CAD build for the part. Positions are in the model's coordinates, mm. Coordinates: 2 decimals unless noted, no trailing zeros. Loops run counter-clockwise (first coordinate to the right, second up) from the corner with the lowest first, then second, coordinate; pieces in that order, holes last. Notation, with made-up numbers: (43.25, 43.25) -> (102.25, 43.25) arc R14 ccw to (102.25, 55.25) -> close; hole circle Ø2 at (-28.5, -39.75). An arc over 180 degrees is marked (long way). Return JSON: item names as keys, results as strings. Group by question number.
(1) Saw through at A-A on z = 2.3. Write the cut outline in (x, y) (3 decimals), then the cut area to 3 significant figures.
(2) Saw through at C-C on y = -30. Write the cut outline in (x, z), then the cut area to 3 significant figures.
(3) Saw through at B-B on y = -72. Write the cut outline in (x, z), then the cut area to 3 significant figures.
(4) Flat gauge pins, fed straight in: pin 1 Ø2 at (x, y) = (44, -75.5) entering from -Z; pin 2 Ø8.5 at (x, y) = (103.24, -70.5) entering from +Z. Where does each tip first touch, or does it go through?
(5) Probe L1, parallel to X at y = -70, z = 0.95; L2, parallel to X at y = -75, z = 1.85; L3, parallel to X at y = -8, z = 0.5. List the from-to ranges inside material, lowest first.
(6) Mould opens along X. For faces 1 (the face through (10.115, -57.366, 1.479)), 2 (the face through (61, -54, 3)), 3 (the face through (98.077, -65.769, 1.521)), 4 (the face through (103.55, -53.293, 1.521)) say: pulls with the +X half, pulls with the -X half, needs draft (parallel to the pull), parting line crosses it, or undercut.
```python
from build123d import *

# Parameters (mm, degrees)
BOSS_EXTRUDE3_DEPTH = 3
SKETCH5_R           = 2.125
SKETCH5_R_2         = 7
CUT_EXTRUDE1_DEPTH  = 10
FILLET1_R           = 10
SKETCH6_R           = 2.125
CUT_EXTRUDE2_DEPTH  = 3


with BuildPart() as part:
    # Sketch4 → Boss-Extrude3 (new body)
    with BuildSketch(Plane.XY):
        Polygon((0, 0), (118.235967878, 0), (118.235967878, -110), (19.395967878, -110), align=None)
    extrude(amount=BOSS_EXTRUDE3_DEPTH)

    # Sketch5 → Cut-Extrude1 (cut)
    with BuildSketch(Plane.XY.offset(3)):
        with Locations((105.235967878, -25)):
            Circle(SKETCH5_R)
        with Locations((15.3749641, -30)):
            Circle(SKETCH5_R)
        with Locations((103.235967878, -70.5)):
            Circle(SKETCH5_R_2)
    extrude(amount=-CUT_EXTRUDE1_DEPTH, mode=Mode.SUBTRACT)

    # Fillet1
    fillet1_edges = [part.edges().sort_by_distance(p)[0] for p in [
        (0, 0, 1.5),
        (118.235967878, 0, 1.5),
        (118.235967878, -110, 1.5),
        (19.395967878, -110, 1.5),
    ]]
    fillet(fillet1_edges, radius=FILLET1_R)

    # Sketch6 → Cut-Extrude2 (cut)
    with BuildSketch(Plane.XY.offset(3)):
        with Locations((105.235967878, -52)):
            Circle(SKETCH6_R)
    extrude(amount=-CUT_EXTRUDE2_DEPTH, mode=Mode.SUBTRACT)


solid = part.part
```
Geometry results:
{
 "1": {"outline": "(2.069, -11.736) -> (17.939, -101.736) arc R10 ccw to (27.787, -110) -> (108.236, -110) arc R10 ccw to (118.236, -100) -> (118.236, -10) arc R10 ccw to (108.236, 0) -> (11.918, 0) arc R10 ccw to start; hole circle Ø4.25 at (15.375, -30); hole circle Ø14 at (103.236, -70.5); hole circle Ø4.25 at (105.236, -52); hole circle Ø4.25 at (105.236, -25)", "area": "11,700 mm²"},
 "2": {"outline": "(5.29, 0) -> (13.25, 0) -> (13.25, 3) -> (5.29, 3) -> close; (17.5, 0) -> (118.24, 0) -> (118.24, 3) -> (17.5, 3) -> close", "area": "326 mm²"},
 "3": {"outline": "(12.7, 0) -> (96.4, 0) -> (96.4, 3) -> (12.7, 3) -> close; (110.07, 0) -> (118.24, 0) -> (118.24, 3) -> (110.07, 3) -> close", "area": "276 mm²"},
 "4": {"pin 1": "z = 0", "pin 2": "through"},
 "5": {"L1": "12.34 to 96.25, 110.22 to 118.24", "L2": "13.22 to 97.87, 108.6 to 118.24", "L3": "2.12 to 118.03"},
 "6": {"face 1": "pulls with the -X half", "face 2": "needs draft", "face 3": "undercut", "face 4": "undercut"}
}
